from build123d import *
from build123d.topology import SkipClean

# Parameters (mm, degrees)
IZIM1_R                     = 8.1
Y_KSEKLIK_EKSTR_ZYON1_DEPTH = 7
RADYUS1_R                   = 1
Y_KSEKLIK_EKSTR_ZYON2_DEPTH = 1
Y_KSEKLIK_EKSTR_ZYON3_DEPTH = 1
IZIM4_W                     = 1.2
IZIM4_H                     = 2.5
Y_KSEKLIK_EKSTR_ZYON4_DEPTH = 3
IZIM5_R                     = 3.4
Y_KSEKLIK_EKSTR_ZYON5_DEPTH = 6.6
IZIM6_R                     = 2.9
Y_KSEKLIK_EKSTR_ZYON6_DEPTH = 1
Y_KSEKLIK_EKSTR_ZYON7_DEPTH = 12
IZIM8_W                     = 13.702328024
IZIM8_H                     = 4.535329086
KES_EKSTR_ZYON1_DEPTH       = 3.5
Y_KSEKLIK_EKSTR_ZYON8_START = 1.9
IZIM9_R                     = 0.75
Y_KSEKLIK_EKSTR_ZYON8_DEPTH = 1.6
Y_KSEKLIK_EKSTR_ZYON9_DEPTH = 1


with BuildPart() as part:
    # Çizim1 → Yükseklik-Ekstrüzyon1 (new body)
    with BuildSketch(Plane.XY):
        Circle(IZIM1_R)
    extrude(amount=Y_KSEKLIK_EKSTR_ZYON1_DEPTH)

    # Radyus1
    radyus1_edges = [part.edges().sort_by_distance(p)[0] for p in [
        (-8.1, 0, 0),
    ]]
    fillet(radyus1_edges, radius=RADYUS1_R)

    # Çizim2 → Yükseklik-Ekstrüzyon2 (add)
    with SkipClean():  # the faces are left unmerged after this step: merging them gives an invalid solid
        with BuildSketch(Plane.XY.offset(7)):
            with BuildLine():
                Line((-5.946427499, 5.5), (5.946427499, 5.5))
                ThreePointArc((5.946427499, 5.5), (8.1, 0), (5.946427499, -5.5))
                Line((5.946427499, -5.5), (-5.946427499, -5.5))
                ThreePointArc((-5.946427499, -5.5), (-8.1, 0), (-5.946427499, 5.5))
            make_face()
        extrude(amount=Y_KSEKLIK_EKSTR_ZYON2_DEPTH)

    # Çizim3 → Yükseklik-Ekstrüzyon3 (add)
    with BuildSketch(Plane.XY.offset(8)):
        with BuildLine():
            Line((-2.5, 5.5), (2.5, 5.5))
            Line((2.5, 5.5), (2.5, 4.673328578))
            ThreePointArc((2.5, 4.673328578), (5.3, 0), (2.5, -4.673328578))
            Line((2.5, -4.673328578), (2.5, -5.5))
            Line((2.5, -5.5), (-2.5, -5.5))
            Line((-2.5, -5.5), (-2.5, -4.673328578))
            ThreePointArc((-2.5, -4.673328578), (-5.3, 0), (-2.5, 4.673328578))
            Line((-2.5, 4.673328578), (-2.5, 5.5))
        make_face()
    extrude(amount=Y_KSEKLIK_EKSTR_ZYON3_DEPTH)

    # Çizim4 → Yükseklik-Ekstrüzyon4 (add)
    with BuildSketch(Plane.XY.offset(8)):
        with Locations((-7.3, 0)):
            Rectangle(IZIM4_W, IZIM4_H)
    extrude(amount=Y_KSEKLIK_EKSTR_ZYON4_DEPTH)

    # Çizim5 → Yükseklik-Ekstrüzyon5 (add)
    with BuildSketch(Plane.XY.offset(9)):
        Circle(IZIM5_R)
    extrude(amount=Y_KSEKLIK_EKSTR_ZYON5_DEPTH)

    # Çizim6 → Yükseklik-Ekstrüzyon6 (add)
    with BuildSketch(Plane.XY.offset(15.6)):
        Circle(IZIM6_R)
    extrude(amount=Y_KSEKLIK_EKSTR_ZYON6_DEPTH)

    # Çizim7 → Yükseklik-Ekstrüzyon7 (add)
    with SkipClean():  # the faces are left unmerged after this step: merging them gives an invalid solid
        with BuildSketch(Plane.XY.offset(16.6)):
            with BuildLine():
                Line((-0.5, 2.856571371), (-0.5, -2.856571371))
                ThreePointArc((-0.5, -2.856571371), (-2.9, 0), (-0.5, 2.856571371))
            make_face()
            with BuildLine():
                Line((0.5, 2.856571371), (0.5, -2.856571371))
                ThreePointArc((0.5, -2.856571371), (2.9, 0), (0.5, 2.856571371))
            make_face()
        extrude(amount=Y_KSEKLIK_EKSTR_ZYON7_DEPTH)

    # Çizim8 → Kes-Ekstrüzyon1 (cut)
    with BuildSketch(Plane.XY.offset(7)):
        with Locations((0.904736513, -7.767664543)):
            Rectangle(IZIM8_W, IZIM8_H)
    extrude(amount=-KES_EKSTR_ZYON1_DEPTH, mode=Mode.SUBTRACT)

    # Çizim9 → Yükseklik-Ekstrüzyon8 (add)
    with BuildSketch(Plane.XY.offset(3.5).offset(Y_KSEKLIK_EKSTR_ZYON8_START)):
        with BuildLine():
            Line((-7.75, -11.5), (7.75, -11.5))
            Line((7.75, -11.5), (7.75, -7.5))
            ThreePointArc((7.75, -7.5), (7.164213562, -6.085786438), (5.75, -5.5))
            Line((5.75, -5.5), (-5.75, -5.5))
            ThreePointArc((-5.75, -5.5), (-7.164213562, -6.085786438), (-7.75, -7.5))
            Line((-7.75, -7.5), (-7.75, -11.5))
        make_face()
        with Locations((0, -8.7)):
            Circle(IZIM9_R, mode=Mode.SUBTRACT)
        with Locations((5.08, -8.7)):
            Circle(IZIM9_R, mode=Mode.SUBTRACT)
        with Locations((-5.08, -8.7)):
            Circle(IZIM9_R, mode=Mode.SUBTRACT)
    extrude(amount=Y_KSEKLIK_EKSTR_ZYON8_DEPTH)

    # Çizim10 → Yükseklik-Ekstrüzyon9 (add)
    with BuildSketch(Plane(origin=(0, 0, 5.4), x_dir=(-1, 0, 0), z_dir=(0, 0, -1))):
        with BuildLine():
            Line((3.53, -12.7), (4.58, -12))
            Line((4.58, -12), (4.58, -15.9))
            ThreePointArc((4.58, -15.9), (4.667867966, -16.112132034), (4.88, -16.2))
            Line((4.88, -16.2), (5.28, -16.2))
            ThreePointArc((5.28, -16.2), (5.492132034, -16.112132034), (5.58, -15.9))
            Line((5.58, -15.9), (5.58, -12))
            Line((5.58, -12), (6.63, -12.7))
            Line((6.63, -12.7), (6.88, -12.7))
            Line((6.88, -12.7), (6.88, -8.7))
            ThreePointArc((6.88, -8.7), (5.08, -6.9), (3.28, -8.7))
            Line((3.28, -8.7), (3.28, -12.7))
            Line((3.28, -12.7), (3.53, -12.7))
        make_face()
        with BuildLine():
            Line((-1.55, -12.7), (-0.5, -12))
            Line((-0.5, -12), (-0.5, -15.9))
            ThreePointArc((-0.5, -15.9), (-0.412132034, -16.112132034), (-0.2, -16.2))
            Line((-0.2, -16.2), (0.2, -16.2))
            ThreePointArc((0.2, -16.2), (0.412132034, -16.112132034), (0.5, -15.9))
            Line((0.5, -15.9), (0.5, -12))
            Line((0.5, -12), (1.55, -12.7))
            Line((1.55, -12.7), (1.8, -12.7))
            Line((1.8, -12.7), (1.8, -8.7))
            ThreePointArc((1.8, -8.7), (0, -6.9), (-1.8, -8.7))
            Line((-1.8, -8.7), (-1.8, -12.7))
            Line((-1.8, -12.7), (-1.55, -12.7))
        make_face()
        with BuildLine():
            Line((-6.63, -12.7), (-5.58, -12))
            Line((-5.58, -12), (-5.58, -15.9))
            ThreePointArc((-5.58, -15.9), (-5.492132034, -16.112132034), (-5.28, -16.2))
            Line((-5.28, -16.2), (-4.88, -16.2))
            ThreePointArc((-4.88, -16.2), (-4.667867966, -16.112132034), (-4.58, -15.9))
            Line((-4.58, -15.9), (-4.58, -12))
            Line((-4.58, -12), (-3.53, -12.7))
            Line((-3.53, -12.7), (-3.28, -12.7))
            Line((-3.28, -12.7), (-3.28, -8.7))
            ThreePointArc((-3.28, -8.7), (-5.08, -6.9), (-6.88, -8.7))
            Line((-6.88, -8.7), (-6.88, -12.7))
            Line((-6.88, -12.7), (-6.63, -12.7))
        make_face()
    extrude(amount=Y_KSEKLIK_EKSTR_ZYON9_DEPTH)


solid = part.part
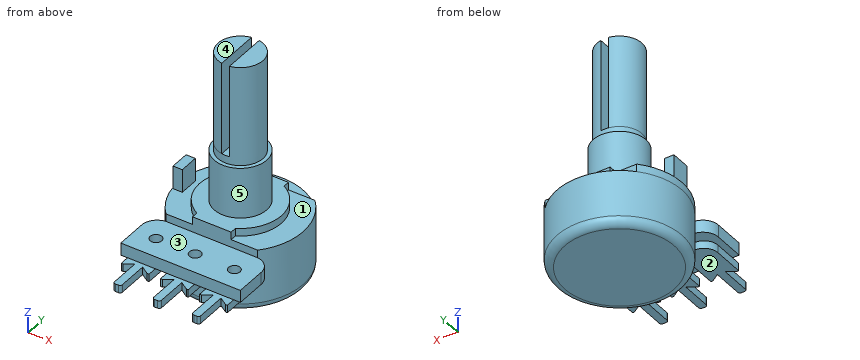
CAD build for the part. Positions are in the model's coordinates, mm. Face numbers are marked on the shaded views. A direction names the side the tool comes from. Coordinates: 2 decimals unless noted, no trailing zeros. Loops run counter-clockwise (first coordinate to the right, second up) from the corner with the lowest first, then second, coordinate; pieces in that order, holes last. Notation, with made-up numbers: (35.25, 56) - (81.25, 56) arc R23 cw to (81.25, 91) - close; hole circle Ø10 at (-34, -2). An arc over 180 degrees is marked (long way). Use one line per item in the form item = value. Start each with the question number.
1) Band-saw the part on B-B (y = 0). Give the cut face in (x, z), and give its area (3 significant figures).
2) Band-saw the part on C-C (z = 10). Give the cut face in (x, y).
3) Band-saw the part on A-A (z = 17.5). Give the cut face in (x, y), and give its area (3 significant figures).
4) Tool access for the marked faces 1, 2, 3, 4 and 5: list every direction of +Z, -Z, +X, -X, +Y, -Y with a clear straight run to the whole face (end or side of a thin tool).
5) Band-saw the part on D-D (z = 13.25). Give the cut face in (x, y), and give its area (3 significant figures).
6) Flat gauge pins, fed straight in: pin 1 (3 mm diameter, centred on x = 5, y = -3.5, fed in from -Z); pin 2 (1 mm diameter, centred on x = 3.5, y = -1.5, fed in from +Z); pin 3 (1.3 mm diameter, centred on x = -2.5, y = 6.5, fed in from +Z); pin 4 (1.8 mm diameter, centred on x = -4.5, y = -15, fed in from +Z). Where does each tip first touch, or does it go through?
7) Drill centre lines: L1, parallel to Z at x = -2, y = -6.5; L2, parallel to Y at x = 0, z = 6.2; L3, parallel to Z at x = 6.5, y = -0.25. Where is each one in solid material? Low to high. Write a range as from..to.
Check values:
q1.outline = (-8.1, 1) arc R1 ccw to (-7.1, 0) - (7.1, 0) arc R1 ccw to (8.1, 1) - (8.1, 8) - (5.3, 8) - (5.3, 9) - (3.4, 9) - (3.4, 15.6) - (2.9, 15.6) - (2.9, 28.6) - (0.5, 28.6) - (0.5, 16.6) - (-0.5, 16.6) - (-0.5, 28.6) - (-2.9, 28.6) - (-2.9, 15.6) - (-3.4, 15.6) - (-3.4, 9) - (-5.3, 9) - (-5.3, 8) - (-6.7, 8) - (-6.7, 11) - (-7.9, 11) - (-7.9, 8) - (-8.1, 8) - close
q1.area = 252 mm2
q2.outline = (-7.9, -1.25) - (-6.7, -1.25) - (-6.7, 1.25) - (-7.9, 1.25) - close; circle Ø6.8 at (0, 0)
q3.outline = (-0.5, -2.86) - (-0.5, 2.86) arc R2.9 ccw to start; (0.5, -2.86) arc R2.9 ccw to (0.5, 2.86) - close
q3.area = 20.6 mm2
q4.face_1 = +Z, +X
q4.face_2 = -Z, +X, -X, -Y
q4.face_3 = +Z, +X, -X, -Y
q4.face_4 = +Z, +X, -X, +Y, -Y
q4.face_5 = +Z
q5.outline = circle Ø6.8 at (0, 0)
q5.area = 36.3 mm2
q6.pin_1 = 0
q6.pin_2 = 15.6
q6.pin_3 = 7
q6.pin_4 = 5.4
q7.L1 = 0..3.5, 5.4..7
q7.L2 = -11.5..-9.45, -7.95..8.1
q7.L3 = 0..8
